from build123d import *

# Parameters (mm, degrees)
F0_R          = 12.5
F2_DEPTH      = 5
F1_W          = 10
F1_H          = 10
F3_DEPTH      = 5.001
F3_DEPTH_BACK = 5.001


with BuildPart() as f2:
    # F0 (on Right) → F2 (new body, symmetric)
    with BuildSketch(Plane.YZ):
        Circle(F0_R)
    extrude(amount=F2_DEPTH, both=True)

    # F1 (on Right) → F3 (cut, two sides)
    with BuildSketch(Plane.YZ) as f3_sk:
        Rectangle(F1_W, F1_H)
    extrude(amount=-F3_DEPTH, mode=Mode.SUBTRACT)
    extrude(f3_sk.sketch, amount=F3_DEPTH_BACK, mode=Mode.SUBTRACT)


solid = f2.part
Geometry: final body of the model. Coordinates: model frame, mm. A direction names the side the tool comes from. Round coordinates to 2 decimals unless told otherwise and drop trailing zeros. Order: outer loops, then holes, each group sorted by start corner. A loop starts at its lowest first (then second) coordinate and runs counter-clockwise, first axis right, second up.
Q1. Section B-B, the plane y = -3.5. Output: boundary loops of the cut face in (x, z).
Result sheet:
outline: (-5, -12) - (5, -12) - (5, -5) - (-5, -5) - close; (-5, 5) - (5, 5) - (5, 12) - (-5, 12) - close
Q2. Mould query, pull axis Z, two halves, no side actions, for faces 1 (the face through (5, -0.2, -5.4)), 2 (the face through (0.07, 11.923, 3.755)), 3 (the face through (0, 5, 0)). Classes: released by +Z, released by -Z, zero draft, split by the parting line, or undercut.
Result sheet:
face 1: zero draft
face 2: split by the parting line
face 3: undercut
Q3. Material intervals for probe 1 along Y at (x, z) = (2, -0.25); probe 2 along Z at (x, y) = (3.5, 0.5); probe 3 along Z at (x, y) = (4, 1.5), sorted ascending.
Result sheet:
probe 1: y = -12.5 to -5, 5 to 12.5
probe 2: z = -12.49 to -5, 5 to 12.49
probe 3: z = -12.41 to -5, 5 to 12.41
Q4. Section C-C, the plane x = -3.25. Output: boundary loops of the cut face in (y, z), and give its area (3 significant figures).
Result sheet:
outline: circle Ø25 at (0, 0); hole (-5, -5) - (5, -5) - (5, 5) - (-5, 5) - close
area: 391 mm2
Q5. Access query for faces 4 (the face through (0, 0, 5)), 5 (the face through (-5, -0.2, -5.4)). Directions: +Z, -Z, +X, -X, +Y, -Y. A direction counts if a zero-diameter tool reaches every point of the face in a straight line with its end or side. Return the directions, or none.
Result sheet:
face 4: +X, -X
face 5: +Z, -Z, -X, +Y, -Y
Q6. Pin query (flat end, axial travel): pin 1 (5 mm diameter, centred on x = -0.5, z = 9, fed in from -Y); pin 2 (4 mm diameter, centred on x = -2, z = 9, fed in from -Y); pin 3 (6 mm diameter, centred on x = -3.5, z = 4.5, fed in from -Y); pin 4 (5 mm diameter, centred on x = 0.5, z = 1, fed in from +Y). Return the tip coordinate at first contact, or that it passes through.
Result sheet:
pin 1: stops at y = -10.68
pin 2: stops at y = -10.36
pin 3: stops at y = -12.41
pin 4: stops at y = 12.5
Q7. Section D-D, the plane z = 8. Output: boundary loops of the cut face in (x, y).
Result sheet:
outline: (-5, -9.6) - (5, -9.6) - (5, 9.6) - (-5, 9.6) - close
Q8. Section A-A, the plane z = 0. Output: boundary loops of the cut face in (x, y).
Result sheet:
outline: (-5, -12.5) - (5, -12.5) - (5, -5) - (-5, -5) - close; (-5, 5) - (5, 5) - (5, 12.5) - (-5, 12.5) - close
